Can you work these out from the model? Positions are in its coordinate system, mm. Give positions to 0.01 mm unless a question says otherwise; leave off trailing zeros. Write each loop counter-clockwise with the first axis right and the second up, starting at its lowest first coordinate (ties: lowest second). Pieces come first, ordered by that corner, then holes.
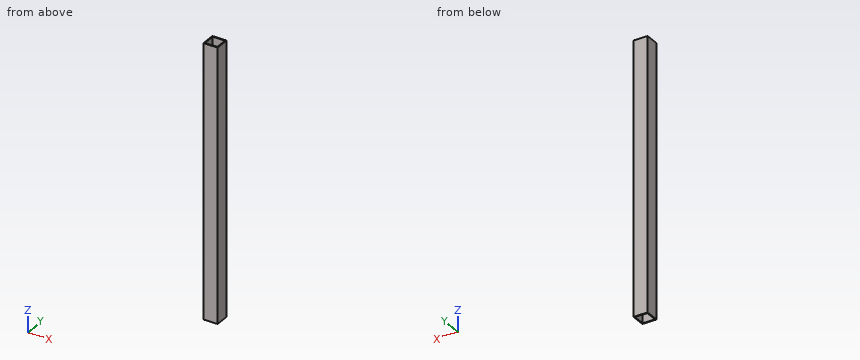
from build123d import *

# Parameters (mm, degrees)
ESBO_O2_W                = 30
ESBO_O2_H                = 30
RESSALTO_EXTRUS_O1_DEPTH = 570
CASCA2_T                 = -2


with BuildPart() as part:
    # Esboço2 → Ressalto-extrusão1 (new body)
    with BuildSketch(Plane.XY):
        with Locations((-79.205213928, 44.662246879)):
            Rectangle(ESBO_O2_W, ESBO_O2_H)
    extrude(amount=RESSALTO_EXTRUS_O1_DEPTH)

    # Casca2
    casca2_openings = [part.faces().sort_by_distance(p)[0] for p in [
        (-79.205213928, 44.662246879, 570),
        (-79.205213928, 44.662246879, 0),
    ]]
    offset(amount=CASCA2_T, openings=casca2_openings, kind=Kind.INTERSECTION)


solid = part.part
(1) Imagine slicing it at B-B, the plane y = 39.25. Write out the boundary of the cut face in (x, z), plus the area to 3 significant figures.
Returned:
outline: (-94.21, 0) - (-92.21, 0) - (-92.21, 570) - (-94.21, 570) - close; (-66.21, 0) - (-64.21, 0) - (-64.21, 570) - (-66.21, 570) - close
area: 2,280 mm2
(2) Imagine slicing it at C-C, the plane z = 225. Write out the boundary of the cut face in (x, y), plus the area to 3 significant figures.
Returned:
outline: (-94.21, 29.66) - (-64.21, 29.66) - (-64.21, 59.66) - (-94.21, 59.66) - close; hole (-92.21, 31.66) - (-66.21, 31.66) - (-66.21, 57.66) - (-92.21, 57.66) - close
area: 224 mm2
(3) Imagine slicing it at A-A, the plane x = -82.25. Write out the boundary of the cut face in (y, z), plus the area to 3 significant figures.
Returned:
outline: (29.66, 0) - (31.66, 0) - (31.66, 570) - (29.66, 570) - close; (57.66, 0) - (59.66, 0) - (59.66, 570) - (57.66, 570) - close
area: 2,280 mm2
(4) If I drill on L1, parallel to X at y = 33, z = 33; L2, parallel to Y at x = -72, z = 72, over which ranges is the centre line in solid material (lowest first)?
Returned:
L1: x = -94.21 to -92.21, -66.21 to -64.21
L2: y = 29.66 to 31.66, 57.66 to 59.66
